Autodesk Fusion 360 part; units mm, degrees
sketch "Sketch1" plane through (0, 0, 0) normal (0, 0, 1) x (1, 0, 0) in component "Base"
  line L0 (0, 0) -> (0, 80)
  line L1 (0, 80) -> (18.5, 80)
  line L2 (18.5, 80) -> (18.5, 35)
  line L3 (18.5, 35) -> (66.5, 35)
  line L4 (66.5, 35) -> (66.5, 0)
  line L5 (66.5, 0) -> (0, 0)
  circle A0 centre (11, 76) radius 1.5
  circle A1 centre (11, 36) radius 1.5
  line L6 (14.5, 80) -> (14.5, 0)
  line L7 (18.5, 35) -> (18.5, 0)
  line L8 (8, 60) -> (8, 48)
  line L9 (8, 48) -> (14.5, 48)
  line L10 (14.5, 48) -> (14.5, 60)
  line L11 (14.5, 60) -> (8, 60)
  dimension "d1" = 80
  dimension "d4" = 3
  dimension "d5" = 11
  dimension "d8" = 0
  dimension "d9" = -40
  dimension "d10" = 4
  dimension "d17" = 14.5
  dimension "d18" = 4
  dimension "d21" = 48
  dimension "d22" = 35
  dimension "d100" = 12
  dimension "d101" = 16
  dimension "d102" = 14.5
  dimension "d103" = 8
extrude "Extrude1" add sketch "Sketch1" along normal blind 3 contours L0 L1 L5 L6 L8 L9 L11 | L1 L2 L5 L6 L7 L10 | L3 L4 L5 L7 in component "Base"
extrude "Extrude2" add sketch "Sketch1" along normal blind 9 contours L1 L2 L5 L6 L7 L10 in component "Base"
chamfer "Chamfer1" distance 2 angle 45 2 edges at (9.6015, 76.5424, 0) (9.6015, 36.5424, 0) in component "Base"
sketch "Sketch7" plane through (18.5, 0, 0) normal (1, 0, 0) x (0, 1, 0) in component "Base"
  line L0 (35, 0) -> (80, 0)
  line L1 (80, 0) -> (80, 9)
  line L2 (80, 9) -> (0, 9)
  line L3 (0, 9) -> (0, 3)
  line L4 (0, 3) -> (35, 3)
  line L5 (35, 3) -> (35, 0)
  line L6 (48, 0) -> (54, 6)
  line L7 (54, 6) -> (60, 0)
  line L8 (48, 0) -> (60, 0)
  dimension "d104" = 45
  dimension "d105" = 45
  dimension "d106" = 20
  dimension "d107" = 12
extrude "Extrude10" cut sketch "Sketch7" against normal blind 4 contours L0 L6 L7 L8 in component "Base"
mirror "Mirror1" about plane through (0, 0, 0) normal (1, 0, 0) of bodies 1 merged in component "Base"
sketch "Sketch2" plane through (0, 0, 3) normal (0, 0, 1) x (-1, 0, 0) in component "Base"
  line L0 (18.5, 0) -> (18.5, -35)
  line L1 (18.5, -35) -> (66.5, -35)
  line L2 (66.5, -35) -> (66.5, 0)
  line L3 (66.5, 0) -> (18.5, 0)
  circle A0 centre (63, -31.5) radius 3.5
  circle A1 centre (26, -31.5) radius 3.5
  circle A2 centre (63, -3.5) radius 3.5
  circle A3 centre (26, -3.5) radius 3.5
  circle A4 centre (63, -31.5) radius 1.35
  circle A5 centre (26, -31.5) radius 1.35
  circle A6 centre (63, -3.5) radius 1.35
  circle A7 centre (26, -3.5) radius 1.35
  dimension "d23" = 7
  dimension "d26" = -37
  dimension "d27" = 28
  dimension "d97" = 2.7
extrude "Extrude3" add sketch "Sketch2" along normal blind 4 contours A1 | A3 | A2 | A0 in component "Base"
sketch "Sketch5" plane through (0, 0, 3) normal (0, 0, 1) x (-1, 0, 0) in component "Base"
  line L0 (-18.5, -35) -> (-18.5, 0)
  line L1 (-18.5, 0) -> (-66.5, 0)
  line L2 (-66.5, 0) -> (-66.5, -35)
  line L3 (-66.5, -35) -> (-18.5, -35)
  circle A0 centre (-31.5949, -16.5277) radius 3.5
  circle A1 centre (-63, -3.5) radius 3.5
  circle A2 centre (-31.5949, -16.5277) radius 1.35
  circle A3 centre (-63, -3.5) radius 1.35
  line L4 (-66.5, -35) -> (-66.5, 0)
  line L5 (-66.5, 0) -> (0, 0)
  dimension "d68" = 7
  dimension "d69" = 7
  dimension "d70" = 34
  dimension "d93" = 2.7
  dimension "d94" = 2.7
extrude "Extrude8" add sketch "Sketch5" along normal blind 4 contours A1 | A0 in component "Base"
component "Base" placed x (1, 0, 0) y (0, 1, 0) z (0, 0, 1) at (0, 0, 0)
equation "d5 = ( 22 / 2 ) * 1 mm"
equation "d17 = ( 29 / 2 ) * 1 mm"
Geometry check sheet. Reference: the model listing, model coordinates, mm. A direction names the side the tool comes from. Give positions to 0.01 mm unless a question says otherwise; leave off trailing zeros. Order: outer loops, then holes, each group sorted by start corner. A loop starts at its lowest first (then second) coordinate and runs counter-clockwise, first axis right, second up.
1. Thickness scan on L1, parallel to Y at x = 11, z = 2.4; L2, parallel to Y at x = -63, z = 4.4; L3, parallel to Y at x = 63, z = 3.9. Record the ranges inside material, lowest first.
2. Access from +Z, -Z, +X, -X, +Y, -Y to the whole of each face (thin tool, end or side, straight path). Record for faces 5 (the face through (-1, 23, 0)), 6 (the face through (-25.95, 33.01, 7)), 7 (the face through (-11, 48, 1)), 8 (the face through (10.788, 34.389, 1.875)), 9 (the face through (63, 4, 3)).
3. Release check for a two-part mould opening along Y. For faces 1 (the face through (-10.788, 37.611, 1.875)), 2 (the face through (17, 57, 3)), 3 (the face through (1, 0, 2)), 4 (the face through (42, 18, 3)) record: pulls with the +Y half, pulls with the -Y half, needs draft (parallel to the pull), parting line crosses it, or undercut.
4. Section check C-C, the plane y = 10. Enter the section's corners in (x, z), and give its area (3 significant figures).
5. Section check B-B, the plane x = 11. Enter the section's corners in (y, z).
6. Gauge pin test, flat ends, axial feed: pin 1 Ø5.5 at (x, y) = (-25.5, 5) entering from +Z; pin 2 Ø14.5 at (x, y) = (-6, 21) entering from +Z; pin 3 Ø0.9 at (x, z) = (-10.5, 1) entering from -Y; pin 4 Ø5 at (y, z) = (47, 4.5) entering from +X. Record the tip position at first contact, or that the pin passes through.
7. Section check A-A, the plane y = 76. Enter the section's corners in (x, z).
8. Section check D-D, the plane x = 39. Enter the section's corners in (y, z).
Values follow:
1. L1: y = 0 to 34.5, 37.5 to 48, 60 to 74.5, 77.5 to 80
1. L2: y = 0 to 2.15, 4.85 to 7, 28 to 30.15, 32.85 to 35
1. L3: y = 0 to 2.15, 4.85 to 7
2. face 5: -Z, +X, -X, +Y, -Y
2. face 6: +Z, -X, +Y, -Y
2. face 7: +Z, -Z
2. face 8: -Z
2. face 9: +Z
3. face 1: undercut
3. face 2: undercut
3. face 3: pulls with the -Y half
3. face 4: needs draft
4. outline: (-66.5, 0) - (66.5, 0) - (66.5, 3) - (18.5, 3) - (18.5, 9) - (14.5, 9) - (14.5, 3) - (-14.5, 3) - (-14.5, 9) - (-18.5, 9) - (-18.5, 3) - (-66.5, 3) - close
4. area: 447 mm2
5. outline: (0, 0) - (32.5, 0) - (34.5, 2) - (34.5, 3) - (0, 3) - close; (37.5, 2) - (39.5, 0) - (48, 0) - (48, 3) - (37.5, 3) - close; (60, 0) - (72.5, 0) - (74.5, 2) - (74.5, 3) - (60, 3) - close; (77.5, 2) - (79.5, 0) - (80, 0) - (80, 3) - (77.5, 3) - close
6. pin 1: stops at z = 7
6. pin 2: stops at z = 3
6. pin 3: stops at y = 0
6. pin 4: stops at x = 18.5
7. outline: (-18.5, 0) - (-14.5, 0) - (-12.5, 2) - (-12.5, 3) - (-14.5, 3) - (-14.5, 9) - (-18.5, 9) - close; (-9.5, 2) - (-7.5, 0) - (7.5, 0) - (9.5, 2) - (9.5, 3) - (-9.5, 3) - close; (12.5, 2) - (14.5, 0) - (18.5, 0) - (18.5, 9) - (14.5, 9) - (14.5, 3) - (12.5, 3) - close
8. outline: (0, 0) - (35, 0) - (35, 3) - (0, 3) - close
